Autodesk Fusion 360 part; units mm, degrees
sketch "Schizzo1" plane through (0, 0, 0) normal (0, 0, 1) x (1, 0, 0)
  line L0 (0, 0) -> (80.3848, 300) construction
  line L1 (80.3848, 300) -> (503.6152, 300) construction
  line L2 (503.6152, 300) -> (584, 0) construction
  line L3 (584, 0) -> (0, 0) construction
  line L4 (53.5898, 200) -> (530.4102, 200) construction
  line L5 (42.8719, 160) -> (541.1281, 160)
  line L6 (64.3078, 240) -> (519.6922, 240)
  line L7 (64.3078, 240) -> (43.6023, 240)
  line L8 (43.6023, 240) -> (22.1663, 160)
  line L9 (22.1663, 160) -> (42.8719, 160)
  line L10 (42.8719, 160) -> (53.5898, 200)
  line L11 (53.5898, 200) -> (57.4204, 200)
  line L12 (57.4204, 200) -> (46.7024, 160)
  line L13 (519.6922, 240) -> (540.3977, 240)
  line L14 (540.3977, 240) -> (561.8337, 160)
  line L15 (561.8337, 160) -> (541.1281, 160)
  line L16 (541.1281, 160) -> (530.4102, 200)
  line L17 (530.4102, 200) -> (526.5796, 200)
  line L18 (526.5796, 200) -> (537.2976, 160)
  line L19 (161.641, 160) -> (167, 180)
  line L20 (167, 180) -> (417, 180)
  line L21 (417, 180) -> (422.359, 160)
  line L22 (292, 180) -> (292, 160) construction
  line L23 (292, 200) -> (252.15, 200)
  line L24 (252.15, 200) -> (252.15, 196.3)
  line L25 (252.15, 196.3) -> (431.85, 196.3)
  line L26 (431.85, 196.3) -> (431.85, 200)
  line L27 (292, 200) -> (431.85, 200)
  dimension "d1" = 75
  dimension "d2" = 75
  dimension "d3" = 584
  dimension "d4" = 300
  dimension "d5" = 200
  dimension "d6" = 40
  dimension "d7" = 40
  dimension "d8" = 3.7
  dimension "d11" = 3.7
  dimension "d12" = 20
  dimension "d13" = 20
  dimension "d14" = 20
  dimension "d15" = 250
  dimension "d20" = 3.7
  dimension "d22" = 139.85
  dimension "d23" = 39.85
extrude "Estrusione1" add sketch "Schizzo1" along normal blind 4 contours L5 L6 L7 L8 L9 L10 L11 L12 L13 L14 L15 L16 L17 L18 L19 L20 L21
fillet "Raccordo1" radius 20 2 edges at (43.6023, 240, 2) (540.3977, 240, 2)
component "Component" placed x (1, 0, 0) y (0, 1, 0) z (0, 0, 1) at (0, 0, 0)
equation "d8 = h - 2 * t"
equation "d11 = h - 2 * t"
equation "d20 = h - 2 * t"
equation "d22 = 140 mm - t"
equation "d23 = 40 mm - t"
Model file for the job. Use its own axes, mm. A direction names the side the tool comes from. Give positions to 0.01 mm unless a question says otherwise; leave off trailing zeros. Order: outer loops, then holes, each group sorted by start corner. A loop starts at its lowest first (then second) coordinate and runs counter-clockwise, first axis right, second up. Notation, with made-up numbers: (86.25, 17) - (133.25, 17) arc R17 ccw to (133.25, 46) - close; hole circle Ø5 at (5, 85). An arc over 180 degrees is marked (long way). Write item = value, one per line. Start each with the question number.
1. Probe line 1 along Y through (x, z) = (277.5, 2.65); line 2 along X through (y, z) = (168, 2.75); line 3 along X through (y, z) = (171, 2.25). List the from-to ranges inside material, lowest first.
2. Cut at A-A, the plane z = 1.45. List the corners of the cut face in (x, y).
3. Cut at C-C, the plane y = 217. List the corners of the cut face in (x, z).
4. Two-plate mould, pull along X, no slides. Class faces 1 (the flat face through (48.156, 179.72, 1.972)), 2 (the flat face through (552.98, 193.04, 1.97)), 3 (the flat face through (288, 209, 4)): pulls with the +X half, pulls with the -X half, needs draft (parallel to the pull), parting line crosses it, or undercut.
5. Cut at B-B, the plane x = 238. List the corners of the cut face in (y, z), and give its area (3 significant figures).
6. Drop a flat-ended pin along its axis: P1, Ø1.2, axis at x = 332, z = 2.5, coming from the -Y side. Give the stop position or say it passes through.
7. Which spindle directions (+Z, -Z, +X, -X, +Y, -Y) get a long thin tool onto all of the face, cutting with end or side? Do faces 4 (the flat face through (31.02, 193.04, 1.97)), 5 (the flat face through (531.864, 180.28, 1.972)). Say none if no direction does.
Taken from the geometry:
q1.line_1 = 180 to 196.3, 200 to 240
q1.line_2 = 24.31 to 45.02, 48.85 to 163.78, 420.22 to 535.15, 538.98 to 559.69
q1.line_3 = 25.11 to 45.82, 49.65 to 164.59, 419.41 to 534.35, 538.18 to 558.89
q2.outline = (22.17, 160) - (42.87, 160) - (53.59, 200) - (57.42, 200) - (46.7, 160) - (161.64, 160) - (167, 180) - (417, 180) - (422.36, 160) - (537.3, 160) - (526.58, 200) - (530.41, 200) - (541.13, 160) - (561.83, 160) - (544.37, 225.18) arc R20 ccw to (525.05, 240) - (58.95, 240) arc R20 ccw to (39.63, 225.18) - close; hole (252.15, 196.3) - (431.85, 196.3) - (431.85, 200) - (252.15, 200) - close
q3.outline = (37.44, 0) - (546.56, 0) - (546.56, 4) - (37.44, 4) - close
q4.face_1 = undercut
q4.face_2 = pulls with the +X half
q4.face_3 = needs draft
q5.outline = (180, 0) - (240, 0) - (240, 4) - (180, 4) - close
q5.area = 240 mm²
q6.P1 = 180
q7.face_4 = +Z, -Z, -X, +Y
q7.face_5 = +Z, -Z
